Here's the drawing with two shaded views (mm, measured from the low corner). I have some questions. A direction names the side the tool comes from. Give positions to 0.01 mm unless a question says otherwise; leave off trailing zeros. Loops run counter-clockwise (first coordinate to the right, second up) from the corner with the lowest first, then second, coordinate; pieces in that order, holes last. Notation, with made-up numbers: M 38.5,81.25 L 76.5,81.25 A32 cw 76.5,110.25 Z; hole C -35.5,84.5 d4. An arc over 180 degrees is marked long. Put each result on its own line as item: value. Start each with the question number.
1) Imagine slicing it at B-B (z = 32). Write out the boundary of the cut face in (x, y).
2) If we mould it in two halves opening along X, with no side actions, what happens to the marked faces 1, 2 and 3? For each: +X half, -X half, draft (parallel to the pull), parting line (faces both ways), or undercut.
3) Please list where these lines run through material, in increasing order: line 1 along Y through (x, z) = (4, 1.5); line 2 along X through (y, z) = (39.55, 9.5); line 3 along X through (y, z) = (20, 1). Write a range as from..to.
4) Imagine slicing it at D-D (x = 5). Write out the boundary of the cut face in (y, z), then the cut area to 3 significant figures.
5) Imagine slicing it at C-C (y = 20). Write out the boundary of the cut face in (x, z).
6) For the marked faces 4, 5 and 6, which set-ups out of +Z, -Z, +X, -X, +Y, -Y let a thin tool reach every point of the face, with its end or its side?
7) For P1, Ø6, axis at x = 4, y = 5, coming from the +Z side; P2, Ø3.5, axis at x = 58, y = 35, coming from the +Z side; P3, Ø21.5, axis at x = 38.5, z = 23, coming from the -Y side; P4, Ø8, axis at x = 10.5, y = 20.5, coming from the +Z side, each with a flat end and sliding along its axis, tell me the tip position at first contact or that it passes through.
8) Imagine slicing it at A-A (x = 15.5). Write out the boundary of the cut face in (y, z).
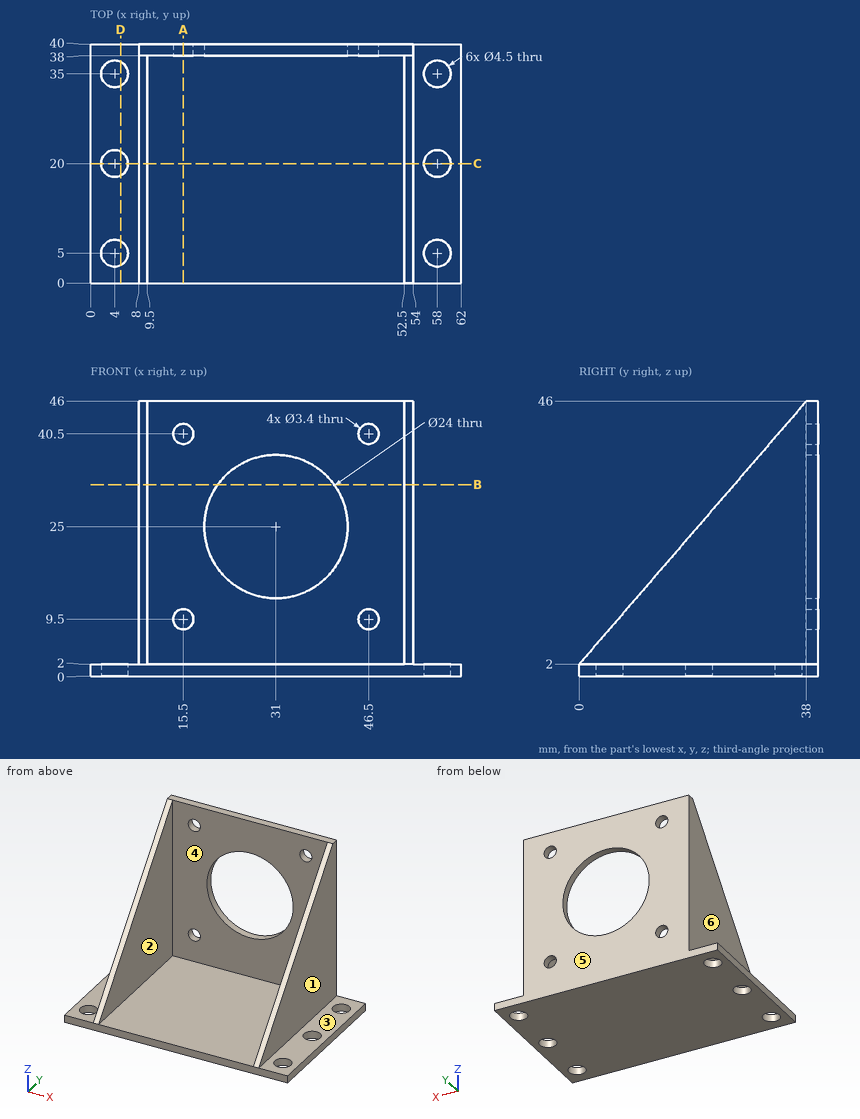
Recorded:
1. outline: M 8,25.91 L 9.5,25.91 L 9.5,38 L 21.25,38 L 21.25,40 L 8,40 Z; M 40.75,38 L 52.5,38 L 52.5,25.91 L 54,25.91 L 54,40 L 40.75,40 Z
2. face 1: +X half
2. face 2: undercut
2. face 3: draft
3. line 1: 0..2.75, 7.25..17.75, 22.25..32.75, 37.25..40
3. line 2: 8..13.8, 17.2..44.8, 48.2..54
3. line 3: 0..1.75, 6.25..55.75, 60.25..62
4. outline: M 0,0 L 2.98,0 L 2.98,2 L 0,2 Z; M 7.02,0 L 17.98,0 L 17.98,2 L 7.02,2 Z; M 22.02,0 L 32.98,0 L 32.98,2 L 22.02,2 Z; M 37.02,0 L 40,0 L 40,2 L 37.02,2 Z
4. area: 55.8 mm²
5. outline: M 0,0 L 1.75,0 L 1.75,2 L 0,2 Z; M 6.25,0 L 55.75,0 L 55.75,2 L 54,2 L 54,25.16 L 52.5,25.16 L 52.5,2 L 9.5,2 L 9.5,25.16 L 8,25.16 L 8,2 L 6.25,2 Z; M 60.25,0 L 62,0 L 62,2 L 60.25,2 Z
6. face 4: +Z, -Y
6. face 5: +Z, -Z, +X, -X, +Y
6. face 6: +Z, -X, +Y, -Y
7. P1: z = 2
7. P2: through
7. P3: y = 38
7. P4: z = 30.22
8. outline: M 0,0 L 40,0 L 40,7.8 L 38,7.8 L 38,2 L 0,2 Z; M 38,11.2 L 40,11.2 L 40,38.8 L 38,38.8 Z; M 38,42.2 L 40,42.2 L 40,46 L 38,46 Z
